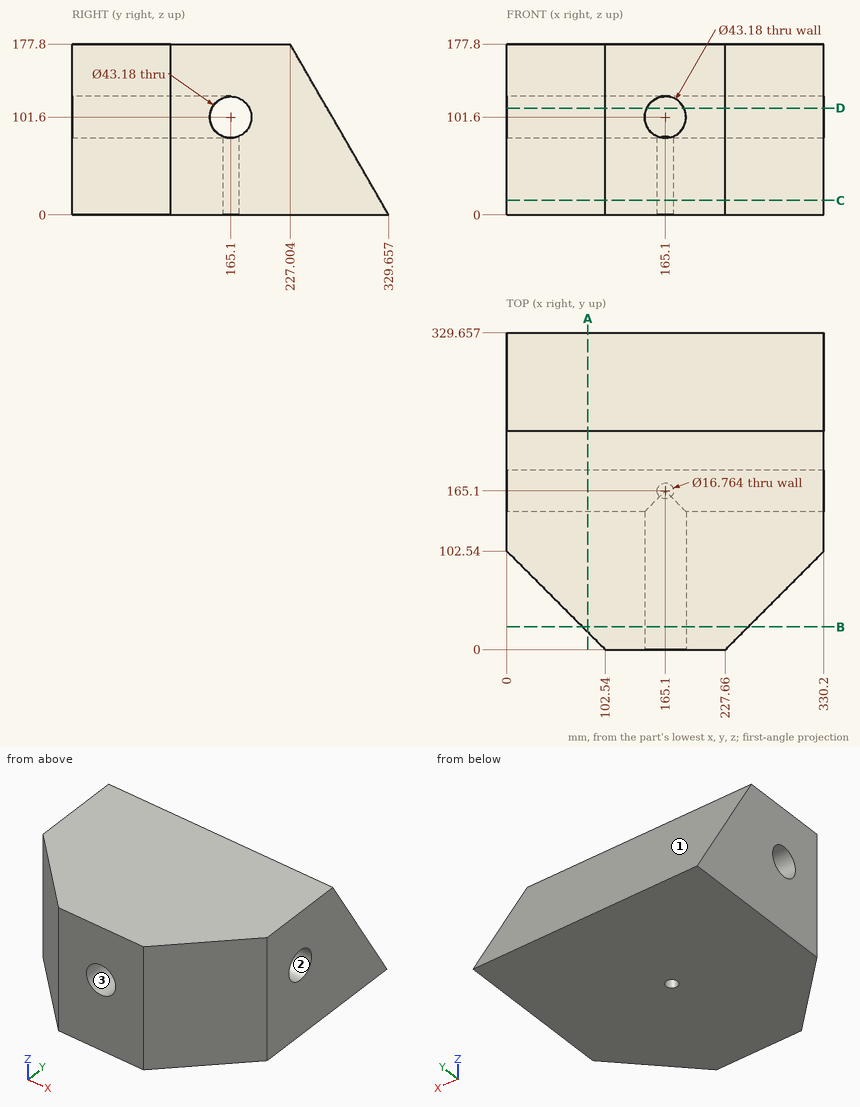
Input: dimensioned drawing with shaded views. Units: mm. Origin: part minimum x, y, z. Give positions to 0.01 mm unless a question says otherwise; leave off trailing zeros. Write each loop counter-clockwise with the first axis right and the second up, starting at its lowest first coordinate (ties: lowest second). Pieces come first, ordered by that corner, then holes. Notation, with made-up numbers: (-14, 89) - (34, 89) arc R17 ccw to (34, 116) - close; hole circle Ø11 at (87.25, 6). An arc over 180 degrees is marked (long way). Write item = value, one per line. Start each with the question number.
1) Cut plane A-A (x = 84.5). Return loops of the section in (y, z) (1 decimal), and give its area (3 significant figures).
2) Cut plane D-D (z = 111). Return loops of the section in (x, y).
3) Cut plane B-B (y = 23.5). Return loops of the section in (x, z), and give its area (3 significant figures).
4) Material intervals for L1, parallel to X at y = 165, z = 50; L2, parallel to Y at x = 49.5, z = 114 (1 decimal); L3, parallel to Y at x = 271.5, z = 118.5 (1 decimal), sorted ascending. Write a range as [from, to].
5) Draft query along Y for the marked faces 1, 2 and 3. Return one class per face: pulls with the +Y half, pulls with the -Y half, needs draft (parallel to the pull), parting line crosses it, or undercut.
6) Cut plane C-C (z = 15). Return loops of the section in (x, y).
7) Pin query (flat end, axial travel): pin 1 (8 mm diameter, centred on x = 233, z = 112.5, fed in from +Y) (1 decimal); pin 2 (10 mm diameter, centred on x = 180.5, z = 104, fed in from -Y); pin 3 (5 mm diameter, centred on y = 61.5, z = 100.5, fed in from -X). Return the tip coordinate at first contact, or that it passes through.
Answers follow:
q1.outline = (18, 0) - (329.7, 0) - (227, 177.8) - (18, 177.8) - close; hole circle Ø43.2 at (165.1, 101.6)
q1.area = 44,800 mm^2
q2.outline = (0, 102.54) - (102.54, 0) - (145.66, 0) - (145.66, 145.66) - (0, 145.66) - close; (0, 184.54) - (330.2, 184.54) - (330.2, 265.57) - (0, 265.57) - close; (184.54, 0) - (227.66, 0) - (330.2, 102.54) - (330.2, 145.66) - (184.54, 145.66) - close
q3.outline = (79.04, 0) - (251.16, 0) - (251.16, 177.8) - (79.04, 177.8) - close; hole circle Ø43.18 at (165.1, 101.6)
q3.area = 29,100 mm^2
q4.L1 = [0, 156.72], [173.48, 330.2]
q4.L2 = [53, 147.4], [182.8, 263.8]
q4.L3 = [43.8, 151.7], [178.5, 261.2]
q5.face_1 = pulls with the +Y half
q5.face_2 = undercut
q5.face_3 = needs draft
q6.outline = (0, 102.54) - (102.54, 0) - (227.66, 0) - (330.2, 102.54) - (330.2, 321) - (0, 321) - close; hole circle Ø16.76 at (165.1, 165.1)
q7.pin_1 = 267
q7.pin_2 = 185.38
q7.pin_3 = 38.54
